The model under review builds one solid part; all positions refer to its coordinate system, in mm. A direction names the side the tool comes from. Round coordinates to 2 decimals unless told otherwise and drop trailing zeros. Order: outer loops, then holes, each group sorted by start corner. A loop starts at its lowest first (then second) coordinate and runs counter-clockwise, first axis right, second up.
```python
from build123d import *

# Parameters (mm, degrees)
SKETCH1_W           = 390
SKETCH1_H           = 756.8
BOSS_EXTRUDE1_DEPTH = 20
SKETCH2_R           = 6.05
BOSS_EXTRUDE2_DEPTH = 10
BOSS_EXTRUDE3_START = 10
SKETCH3_R           = 6.05
BOSS_EXTRUDE3_DEPTH = 10
CHAMFER1_SIZE       = 10
BOSS_EXTRUDE4_DEPTH = 50
SKETCH5_W           = 30
SKETCH5_H           = 160
CUT_EXTRUDE1_DEPTH  = 131
CHAMFER2_SIZE       = 10


with BuildPart() as part:
    # Sketch1 → Boss-Extrude1 (new body)
    with BuildSketch(Plane.XY):
        with Locations((147.890593688, -358.84384058)):
            Rectangle(SKETCH1_W, SKETCH1_H)
    extrude(amount=BOSS_EXTRUDE1_DEPTH)

    # Sketch2 → Boss-Extrude2 (add)
    with BuildSketch(Plane(origin=(0, 19.55615942, 0), x_dir=(1, 0, 0), z_dir=(0, 1, 0))):
        with Locations(Location((329.77827945, -10, 0), (0, 0, 90))):
            Circle(SKETCH2_R)
    extrude(amount=BOSS_EXTRUDE2_DEPTH)

    # Sketch3 → Boss-Extrude3 (add)
    with BuildSketch(Plane.XZ.offset(737.24384058).offset(BOSS_EXTRUDE3_START)):
        with Locations(Location((329.77827945, 10, 0), (0, 0, 270))):
            Circle(SKETCH3_R)
    extrude(amount=-BOSS_EXTRUDE3_DEPTH)

    # Chamfer1
    # the kernel refuses this chamfer: 10 mm, written as the material it takes off along each edge
    with BuildSketch(Plane(origin=(368.607423567, -737.24384058, 0), x_dir=(0, 0.9996219169112968, -0.027495876610586487), z_dir=(-1, 0, 0))) as chamfer1_piece_1_section:
        Polygon((CHAMFER1_SIZE * 0.999621916911, -CHAMFER1_SIZE * 0.0274958766106), (-CHAMFER1_SIZE * 0.0274958766106, -CHAMFER1_SIZE * 0.999621916911), (0, 0), align=None)
    chamfer1_piece_1 = extrude(amount=441.433659759, mode=Mode.PRIVATE)
    chamfer1_piece_1 = chamfer1_piece_1 - Plane(origin=(329.77827945, -733.933944157, 10), x_dir=(0, 0, -1), z_dir=(0, -1, 0)) * Cylinder(6.05, 923, mode=Mode.PRIVATE)
    add(chamfer1_piece_1, mode=Mode.SUBTRACT)
    with BuildSketch(Plane(origin=(-47.109406312, -762.960670459, 0), x_dir=(-0.027495876610586317, 0, 0.9996219169112968), z_dir=(0, 1, 0)), Plane(origin=(342.890593688, 45.2729893, 20), x_dir=(-0.9996219169112968, 0, 0.027495876610586282), z_dir=(0, -1, 0))) as chamfer1_piece_2:
        Polygon((CHAMFER1_SIZE * 0.999621916911, CHAMFER1_SIZE * 0.0274958766106), (-CHAMFER1_SIZE * 0.0274958766106, CHAMFER1_SIZE * 0.999621916911), (0, 0), align=None)
    extrude(amount=808.233659759, mode=Mode.SUBTRACT)
    with BuildSketch(Plane(origin=(-72.826236192, 19.55615942, 0), x_dir=(0, 0.027495876610586317, 0.9996219169112968), z_dir=(1, 0, 0))) as chamfer1_piece_3_section:
        Polygon((CHAMFER1_SIZE * 0.999621916911, CHAMFER1_SIZE * 0.0274958766106), (-CHAMFER1_SIZE * 0.0274958766106, CHAMFER1_SIZE * 0.999621916911), (0, 0), align=None)
    chamfer1_piece_3 = extrude(amount=441.433659759, mode=Mode.PRIVATE)
    chamfer1_piece_3 = chamfer1_piece_3 - Plane(origin=(329.77827945, 16.24626296, 10), x_dir=(0, 0, -1), z_dir=(0, -1, 0)) * Cylinder(6.05, 923, mode=Mode.PRIVATE)
    add(chamfer1_piece_3, mode=Mode.SUBTRACT)
    with BuildSketch(Plane(origin=(342.890593688, 45.2729893, 0), x_dir=(-0.9996219169112968, 0, -0.027495876610586334), z_dir=(0, -1, 0)), Plane(origin=(-47.109406312, -762.960670459, 20), x_dir=(-0.027495876610586317, 0, -0.9996219169112968), z_dir=(0, 1, 0))) as chamfer1_piece_4:
        Polygon((CHAMFER1_SIZE * 0.999621916911, -CHAMFER1_SIZE * 0.0274958766106), (-CHAMFER1_SIZE * 0.0274958766106, -CHAMFER1_SIZE * 0.999621916911), (0, 0), align=None)
    extrude(amount=808.233659759, mode=Mode.SUBTRACT)
    with BuildSketch(Plane(origin=(368.607423567, -737.24384058, 20), x_dir=(0, 0.9996219169112968, 0.02749587661058643), z_dir=(-1, 0, 0))) as chamfer1_piece_5_section:
        Polygon((CHAMFER1_SIZE * 0.999621916911, CHAMFER1_SIZE * 0.0274958766106), (-CHAMFER1_SIZE * 0.0274958766106, CHAMFER1_SIZE * 0.999621916911), (0, 0), align=None)
    chamfer1_piece_5 = extrude(amount=441.433659759, mode=Mode.PRIVATE)
    chamfer1_piece_5 = chamfer1_piece_5 - Plane(origin=(329.77827945, -733.933944133, 10), x_dir=(0, 0, -1), z_dir=(0, -1, 0)) * Cylinder(6.05, 923, mode=Mode.PRIVATE)
    add(chamfer1_piece_5, mode=Mode.SUBTRACT)
    with BuildSketch(Plane(origin=(-72.826236192, 19.55615942, 20), x_dir=(0, 0.027495876610586317, -0.9996219169112968), z_dir=(1, 0, 0))) as chamfer1_piece_6_section:
        Polygon((CHAMFER1_SIZE * 0.999621916911, -CHAMFER1_SIZE * 0.0274958766106), (-CHAMFER1_SIZE * 0.0274958766106, -CHAMFER1_SIZE * 0.999621916911), (0, 0), align=None)
    chamfer1_piece_6 = extrude(amount=441.433659759, mode=Mode.PRIVATE)
    chamfer1_piece_6 = chamfer1_piece_6 - Plane(origin=(329.77827945, 16.246262993, 10), x_dir=(0, 0, -1), z_dir=(0, -1, 0)) * Cylinder(6.05, 923, mode=Mode.PRIVATE)
    add(chamfer1_piece_6, mode=Mode.SUBTRACT)

    # Sketch4 → Boss-Extrude4 (add)
    with BuildSketch(Plane.XY.offset(20)):
        Polygon((12.890593688, -358.84384058), (12.890593688, -258.84384058), (-37.109406312, -258.84384058), (-37.109406312, -458.84384058), (12.890593688, -458.84384058), align=None)
    extrude(amount=BOSS_EXTRUDE4_DEPTH)

    # Sketch5 → Cut-Extrude1 (cut)
    with BuildSketch(Plane.ZY.offset(37.109406312)):
        with Locations((35, -358.84384058)):
            Rectangle(SKETCH5_W, SKETCH5_H)
    extrude(amount=-CUT_EXTRUDE1_DEPTH, mode=Mode.SUBTRACT)

    # Chamfer2
    chamfer2_edges = [part.edges().sort_by_distance(p)[0] for p in [
        (-37.109406312, -458.84384058, 45),
        (12.890593688, -458.84384058, 45),
        (12.890593688, -258.84384058, 45),
        (-37.109406312, -258.84384058, 45),
        (-12.109406312, -458.84384058, 70),
        (12.890593688, -358.84384058, 70),
        (-12.109406312, -258.84384058, 70),
        (-37.109406312, -358.84384058, 70),
    ]]
    chamfer(chamfer2_edges, length=CHAMFER2_SIZE)


solid = part.part
```
(1) Consider section A-A (z = 37). Write out the cut boundary in (x, y).
Data:
outline: (-37.11, -448.84) - (-27.11, -458.84) - (2.89, -458.84) - (12.89, -448.84) - (12.89, -438.84) - (-37.11, -438.84) - close; (-37.11, -278.84) - (12.89, -278.84) - (12.89, -268.84) - (2.89, -258.84) - (-27.11, -258.84) - (-37.11, -268.84) - close
(2) Draft analysis for pull direction Y (two halves, no side actions). For faces 4 (the flat face through (12.891, -365.9, 50.3)), 5 (the flat face through (-12, -458.844, 40)), 6 (the flat face through (-12, -278.844, 35)), state which applies: pulls with the +Y half, pulls with the -Y half, needs draft (parallel to the pull), parting line crosses it, or undercut.
Data:
face 4: needs draft
face 5: pulls with the -Y half
face 6: undercut
(3) To check wall thickness, follow probe 1 along Z at (x, y) = (33.5, -202.5); probe 2 along Z at (x, y) = (-29, -433.5); probe 3 along Y at (x, z) = (-29.5, 30). State the ranges of each line that lie inside material, in increasing order.
Data:
probe 1: z = 0 to 20
probe 2: z = 0 to 20, 50 to 68.11
probe 3: y = -456.45 to -438.84, -278.84 to -261.23
(4) Consider section C-C (y = -509.5). Write out the cut boundary in (x, z).
Data:
outline: (-47.11, 10) - (-37.11, 0) - (332.89, 0) - (342.89, 10) - (332.89, 20) - (-37.11, 20) - close
(5) For faces 1 (the flat face through (-12, -438.844, 35)), 2 (the flat face through (-12, -258.844, 40)), 3 (the flat face through (-37.109, -351.8, 50.3)), list the 3-axis set-ups (+Z, -Z, +X, -X, +Y, -Y) from which the entire face can be reached by the end or side of a thin tool; tool diameter is ignored.
Data:
face 1: +X, -X
face 2: +Z, +X, -X, +Y
face 3: +Z, -X, +Y, -Y
(6) Insertion check: pin 1 (12 mm diameter, centred on x = 36, z = 21.5, fed in from -Y); pin 2 (9 mm diameter, centred on x = 0, z = 31, fed in from -Y); pin 3 (12 mm diameter, centred on x = 175, y = -72.5, fed in from +Z). Each pin has a flat end and moves straight along its axis. Give the tip position at first contact, or say it passes through.
Data:
pin 1: stops at y = -731.74
pin 2: stops at y = -458.84
pin 3: stops at z = 20
(7) Consider section B-B (x = 87). Write out the cut boundary in (y, z), and give its area (3 significant figures).
Data:
outline: (-737.24, 10) - (-727.24, 0) - (9.56, 0) - (19.56, 10) - (9.56, 20) - (-727.24, 20) - close
area: 14,900 mm2
